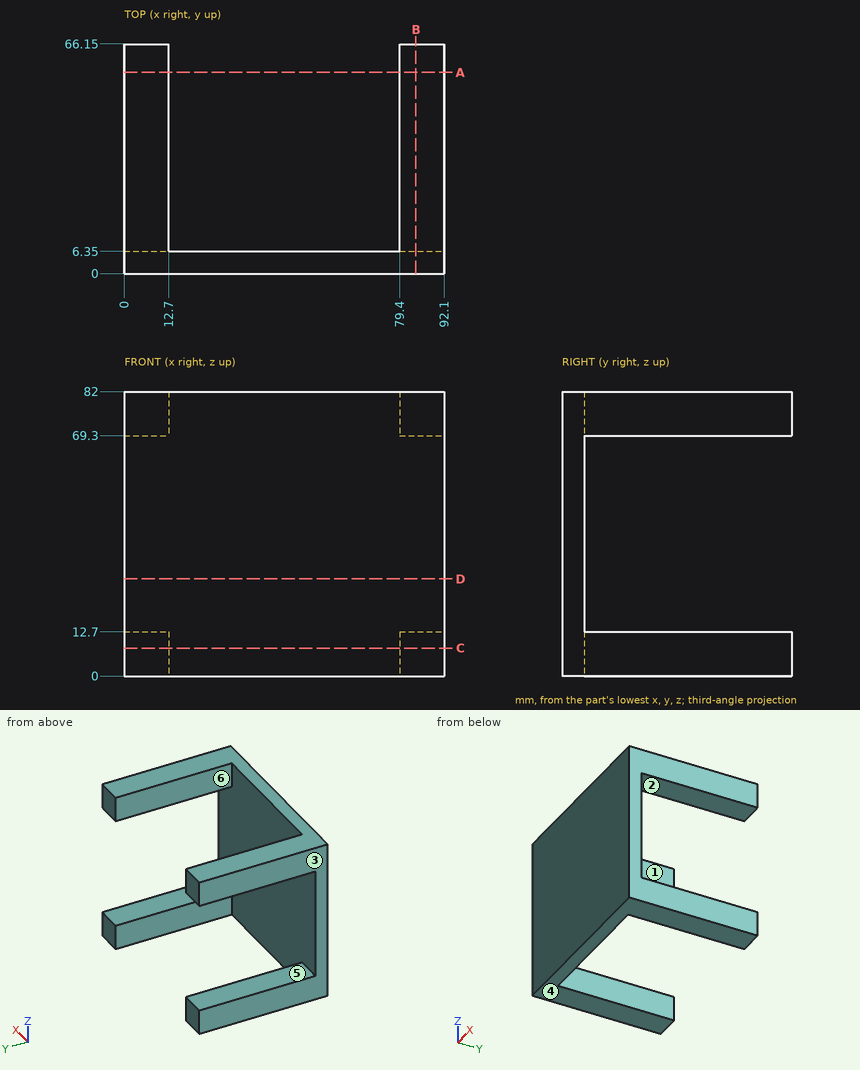
For this review, use the dimensioned drawing (mm, ordinates from the lowest corner) and the shaded views. A direction names the side the tool comes from. Give positions to 0.01 mm unless a question says otherwise; leave off trailing zeros. Order: outer loops, then holes, each group sorted by start corner. A loop starts at its lowest first (then second) coordinate and runs counter-clockwise, first axis right, second up. Notation, with made-up numbers: (85.5, 79) -> (105.5, 79) arc R18 ccw to (105.5, 104) -> close; hole circle Ø9 at (75.25, 85). An arc over 180 degrees is marked (long way). Write item = value, one per line. Start each with the question number.
(1) Draft analysis for pull direction Z (two halves, no side actions). For the marked faces 4, 5 and 6, state which applies: +Z half, -Z half, draft (parallel to the pull), parting line (faces both ways), or undercut.
(2) Take a section at C-C (z = 8). Write out the cut boundary in (x, y), plus the area to 3 significant figures.
(3) Take a section at A-A (y = 58). Write out the cut boundary in (x, z).
(4) Take a section at D-D (z = 28). Write out the cut boundary in (x, y).
(5) Take a section at B-B (x = 84). Write out the cut boundary in (y, z), plus the area to 3 significant figures.
(6) For L1, parallel to X at y = 31, z = 73; L2, parallel to Y at x = 13.5, z = 32; L3, parallel to Z at x = 81.5, y = 50.5, list the stretches that pass through material, from the lowest coordinate up. Write a range as from..to.
(7) For pin 1 Ø2 at (x, z) = (37, 17.5) entering from +Y, flat-tipped, find the tip position at first contact; note if it passes through.
(8) Tool access review of the marked faces 1, 2 and 3: name each direction out of +Z, -Z, +X, -X, +Y, -Y from which nothing blocks a thin tool from reaching the whole face with its end or side.
Returned:
q1.face_4 = -Z half
q1.face_5 = undercut
q1.face_6 = draft
q2.outline = (0, 0) -> (92.1, 0) -> (92.1, 66.15) -> (79.4, 66.15) -> (79.4, 6.35) -> (12.7, 6.35) -> (12.7, 66.15) -> (0, 66.15) -> close
q2.area = 2,100 mm²
q3.outline = (0, 0) -> (12.7, 0) -> (12.7, 12.7) -> (0, 12.7) -> close; (0, 69.3) -> (12.7, 69.3) -> (12.7, 82) -> (0, 82) -> close; (79.4, 0) -> (92.1, 0) -> (92.1, 12.7) -> (79.4, 12.7) -> close; (79.4, 69.3) -> (92.1, 69.3) -> (92.1, 82) -> (79.4, 82) -> close
q4.outline = (0, 0) -> (92.1, 0) -> (92.1, 6.35) -> (0, 6.35) -> close
q5.outline = (0, 0) -> (66.15, 0) -> (66.15, 12.7) -> (6.35, 12.7) -> (6.35, 69.3) -> (66.15, 69.3) -> (66.15, 82) -> (0, 82) -> close
q5.area = 2,040 mm²
q6.L1 = 0..12.7, 79.4..92.1
q6.L2 = 0..6.35
q6.L3 = 0..12.7, 69.3..82
q7.pin_1 = 6.35
q8.face_1 = +Z, -Z, +Y
q8.face_2 = +X, -X, +Y
q8.face_3 = +Z, -Z, -X, +Y, -Y
